Geometry check sheet. Reference: the model listing, model coordinates, mm. Coordinates: 2 decimals unless noted, no trailing zeros. Order: outer loops, then holes, each group sorted by start corner. A loop starts at its lowest first (then second) coordinate and runs counter-clockwise, first axis right, second up.
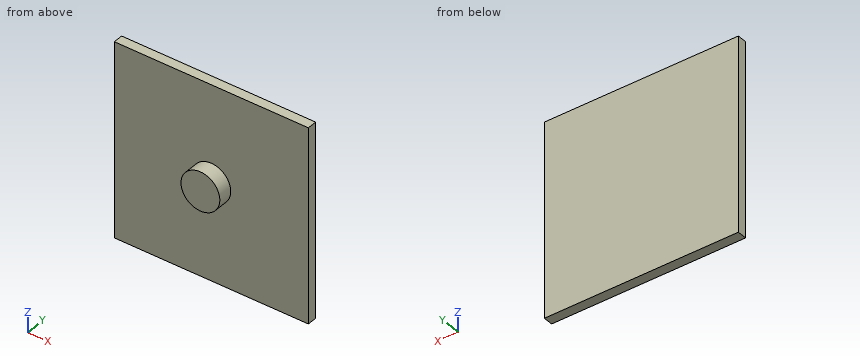
Autodesk Inventor part; units mm, degrees
ref_plane "YZ Plane" through (0, 0, 0) normal (1, 0, 0) x (0, 1, 0)
ref_plane "XZ Plane" through (0, 0, 0) normal (0, 1, 0) x (-1, 0, 0)
ref_plane "XY Plane" through (0, 0, 0) normal (0, 0, 1) x (1, 0, 0)
sketch "Sketch46" plane through (0, 0, 0) normal (0, 1, 0) x (-1, 0, 0)
  circle A0 centre (0, 0) radius 4
  dimension "d158" = 8
extrude "Extrusion35" add sketch "Sketch46" along normal blind 3
sketch "Sketch47" plane through (0, 3, 0) normal (0, 1, 0) x (1, 0, 0)
  line L0 (-20, 20) -> (20, 20)
  line L1 (20, 20) -> (20, -20)
  line L2 (20, -20) -> (-20, -20)
  line L3 (-20, -20) -> (-20, 20)
  line L4 (-20, 20) -> (20, -20) construction
  line L5 (20, 20) -> (-20, -20) construction
  point P0 (0, 0)
  dimension "d161" = 40
  dimension "d162" = 40
extrude "Extrusion36" add sketch "Sketch47" along normal blind 2
properties part number "Front_base"
Item 1: Thickness scan on line 1 along Y through (x, z) = (14, -4); line 2 along Z through (x, y) = (-1, 2.8); line 3 along X through (y, z) = (2.2, 2). Record the ranges inside material, lowest first.
Item 2: Sectioned sample at A-A (x = 0). Record the cut outline in (y, z), and give its area (3 significant figures).
Item 3: Sectioned sample at D-D (x = -9). Record the cut outline in (y, z), and give its area (3 significant figures).
Item 4: Sectioned sample at B-B (z = 0). Record the cut outline in (x, y).
Item 5: Depth check by flat-ended pin: P1, Ø1, axis at x = -1.5, y = 1, coming from the -Z side; P2, Ø10, axis at x = 13, z = 12, coming from the -Y side. Enter the tip coordinate at first touch or a pass-through.
Item 6: Sectioned sample at C-C (y = 2.4). Record the cut outline in (x, z).
Geometry check:
1. line 1: y = 3 to 5
1. line 2: z = -3.87 to 3.87
1. line 3: x = -3.46 to 3.46
2. outline: (0, -4) - (3, -4) - (3, -20) - (5, -20) - (5, 20) - (3, 20) - (3, 4) - (0, 4) - close
2. area: 104 mm2
3. outline: (3, -20) - (5, -20) - (5, 20) - (3, 20) - close
3. area: 80.0 mm2
4. outline: (-20, 3) - (-4, 3) - (-4, 0) - (4, 0) - (4, 3) - (20, 3) - (20, 5) - (-20, 5) - close
5. P1: stops at z = -3.87
5. P2: stops at y = 3
6. outline: circle Ø8 at (0, 0)
